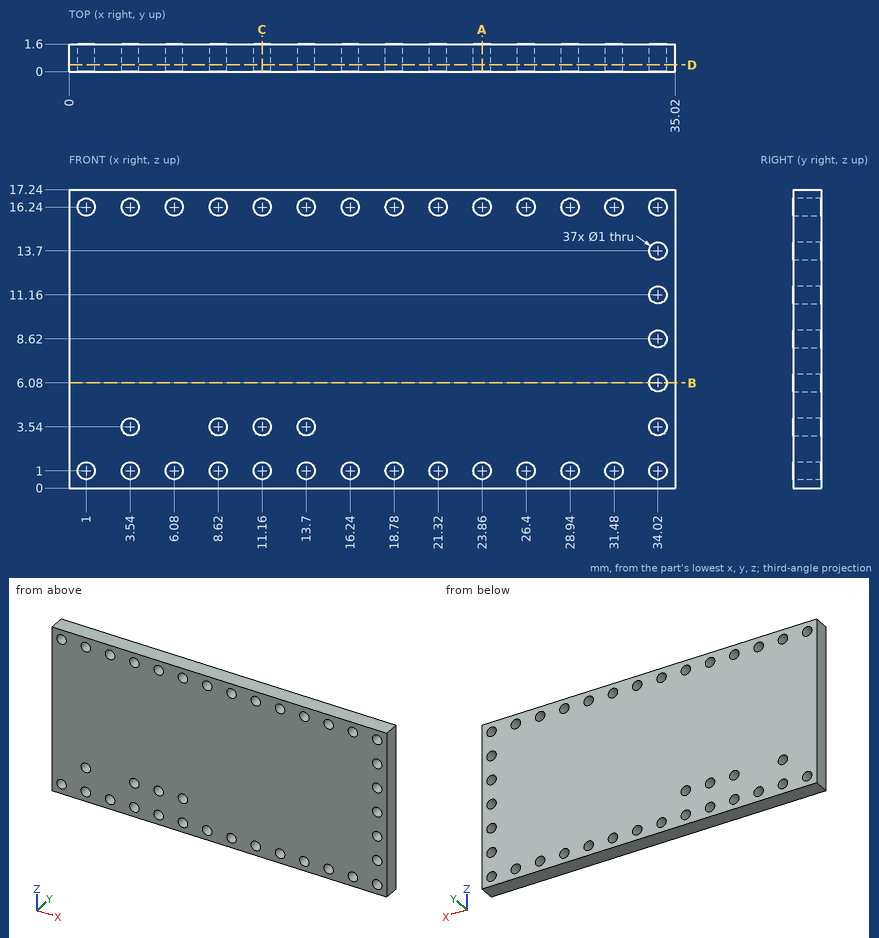
The drawing under review shows one solid part. Ordinate dimensions are in mm from its lowest x, y, z. Coordinates: 2 decimals unless noted, no trailing zeros. Loops run counter-clockwise (first coordinate to the right, second up) from the corner with the lowest first, then second, coordinate; pieces in that order, holes last. Notation, with made-up numbers: (-8.75, -12) - (5.25, -12) arc R13 cw to (5.25, -2) - close; hole circle Ø4 at (-22.5, 1). An arc over 180 degrees is marked (long way). Use CSV: the item, a comma, the result in double quotes. Start each with the question number.
1. Add section C-C on x = 11.16. Give the boundary of the cut face in (y, z).
2. To check wall thickness, follow probe 1 along X at (y, z) = (1.1, 3.54); probe 2 along Z at (x, y) = (11, 1.5); probe 3 along Z at (x, y) = (11.5, 1.3). State the ranges of each line that lie inside material, in increasing order.
3. Add section A-A on x = 23.86. Give the boundary of the cut face in (y, z).
4. Add section B-B on z = 6.08. Give the boundary of the cut face in (x, y), plus the area to 3 significant figures.
5. Add section D-D on y = 0.4. Count the separate pieces of the cut face and the enclosed holes in it, plus the area to 3 significant figures.
Resolved:
1,outline,"(0, 0) - (1.6, 0) - (1.6, 0.5) - (0, 0.5) - close; (0, 1.5) - (1.6, 1.5) - (1.6, 3.04) - (0, 3.04) - close; (0, 4.04) - (1.6, 4.04) - (1.6, 15.74) - (0, 15.74) - close; (0, 16.74) - (1.6, 16.74) - (1.6, 17.24) - (0, 17.24) - close"
2,probe 1,"0 to 3.04, 4.04 to 8.12, 9.12 to 10.66, 11.66 to 13.2, 14.2 to 33.52, 34.52 to 35.02"
2,probe 2,"0 to 0.53, 1.47 to 3.07, 4.01 to 15.77, 16.71 to 17.24"
2,probe 3,"0 to 0.63, 1.37 to 3.17, 3.91 to 15.87, 16.61 to 17.24"
3,outline,"(0, 0) - (1.6, 0) - (1.6, 0.5) - (0, 0.5) - close; (0, 1.5) - (1.6, 1.5) - (1.6, 15.74) - (0, 15.74) - close; (0, 16.74) - (1.6, 16.74) - (1.6, 17.24) - (0, 17.24) - close"
4,outline,"(0, 0) - (33.52, 0) - (33.52, 1.6) - (0, 1.6) - close; (34.52, 0) - (35.02, 0) - (35.02, 1.6) - (34.52, 1.6) - close"
4,area,"54.4 mm2"
5,separate pieces,"1"
5,enclosed holes,"37"
5,area,"575 mm2"
